Input: part model. Units: mm. Frame: model coordinates. A direction names the side the tool comes from. Round coordinates to 2 decimals unless told otherwise and drop trailing zeros. Write each loop counter-clockwise with the first axis right and the second up, starting at its lowest first coordinate (ties: lowest second). Pieces come first, ordered by that corner, then holes. Notation, with made-up numbers: (-33.75, 75.5) -> (3.25, 75.5) arc R35 cw to (3.25, 107.5) -> close; hole circle Ø5 at (62.5, -38.5). An arc over 180 degrees is marked (long way). Write item = value, one per line. Start each with the question number.
```python
from build123d import *

# Parameters (mm, degrees)
SKETCH1_W           = 11
SKETCH1_H           = 76
BOSS_EXTRUDE1_DEPTH = 7
SKETCH4_R           = 2.5
SKETCH5_W           = 3
SKETCH5_H           = 3
BOSS_EXTRUDE2_DEPTH = 4.5
SKETCH6_W           = 2
SKETCH6_H           = 4
CUT_EXTRUDE2_DEPTH  = 2
BOSS_EXTRUDE3_DEPTH = 3
SKETCH10_W          = 11
SKETCH10_H          = 3.5
CUT_EXTRUDE5_DEPTH  = 35
CUT_EXTRUDE6_REACH  = 41.912
SKETCH11_R          = 2.5
SKETCH12_W          = 11
SKETCH12_H          = 2.25
CUT_EXTRUDE9_DEPTH  = 5
CUT_EXTRUDE10_REACH = 41.58
BOSS_EXTRUDE4_START = 2.5
SKETCH15_R          = 4
SKETCH15_R_2        = 2.5
BOSS_EXTRUDE4_DEPTH = 2.5


with BuildPart() as part:
    # Sketch1 → Boss-Extrude1 (new body)
    with BuildSketch(Plane(origin=(0, 0, 0), x_dir=(1, 0, 0), z_dir=(0, 1, 0))):
        Rectangle(SKETCH1_W, SKETCH1_H)
    extrude(amount=BOSS_EXTRUDE1_DEPTH)

    # Cut-Sweep2: sweep along a path in Sketch3
    with BuildLine(Plane.ZY) as cut_sweep2_path:
        Line((-38, 3.5), (28, 3.5))
        ThreePointArc((28, 3.5), (30.121320344, 2.621320344), (31, 0.5))
        Line((31, 0.5), (31, 0))
    # Sketch4 → Cut-Sweep2 (sweep, cut)
    with BuildSketch(Plane(origin=(0, 0, -38), x_dir=(-1, 0, 0), z_dir=(0, 0, -1))):
        with Locations((0, 3.5)):
            Circle(SKETCH4_R)
    sweep(path=cut_sweep2_path.line, mode=Mode.SUBTRACT)

    # Sketch5 → Boss-Extrude2 (add)
    with BuildSketch(Plane.ZY.offset(5.5)):
        with Locations((31.5, 3.5)):
            Rectangle(SKETCH5_W, SKETCH5_H)
    boss_extrude2 = extrude(amount=BOSS_EXTRUDE2_DEPTH)

    # Mirror1: Boss-Extrude2 across plane
    add(boss_extrude2.mirror(Plane.ZY))

    # Sketch6 → Cut-Extrude2 (cut)
    with BuildSketch(Plane.XY.offset(33)):
        with Locations((-7.25, 4)):
            Rectangle(SKETCH6_W, SKETCH6_H)
    cut_extrude2 = extrude(amount=-CUT_EXTRUDE2_DEPTH, mode=Mode.SUBTRACT)

    # Mirror2: Cut-Extrude2 across plane
    add(cut_extrude2.mirror(Plane.ZY), mode=Mode.SUBTRACT)

    # Sketch7 → Boss-Extrude3 (add)
    with BuildSketch(Plane(origin=(0, 5, 0), x_dir=(1, 0, 0), z_dir=(0, 1, 0))):
        Polygon((-10, -30), (-5.5, -25.5), (-5.5, -30), align=None)
    boss_extrude3 = extrude(amount=-BOSS_EXTRUDE3_DEPTH)

    # Mirror3: Boss-Extrude3 across plane
    add(boss_extrude3.mirror(Plane.ZY))

    # Sketch10 → Cut-Extrude5 (cut)
    with BuildSketch(Plane(origin=(0, 0, -38), x_dir=(-1, 0, 0), z_dir=(0, 0, -1))):
        with Locations((0, 3.5)):
            Rectangle(SKETCH10_W, SKETCH10_H)
    extrude(amount=-CUT_EXTRUDE5_DEPTH, mode=Mode.SUBTRACT)

    # Sketch11 → Cut-Extrude6 (cut, up to next)
    with BuildSketch(Plane(origin=(0, 7, 0), x_dir=(1, 0, 0), z_dir=(0, 1, 0)), mode=Mode.PRIVATE) as cut_extrude6_sk1:
        with Locations(Location((0, 13, 0), (0, 0, 270))):
            Circle(SKETCH11_R)
    cut_extrude6_tool1 = extrude(cut_extrude6_sk1.sketch, amount=-CUT_EXTRUDE6_REACH, mode=Mode.PRIVATE) & part.part
    add(cut_extrude6_tool1.solids().sort_by_distance((0, 7, -13))[0], mode=Mode.SUBTRACT)

    # Sketch12 → Cut-Extrude9 (cut)
    with BuildSketch(Plane.XY.offset(38)):
        with Locations((0, 5.875)):
            Rectangle(SKETCH12_W, SKETCH12_H)
    extrude(amount=-CUT_EXTRUDE9_DEPTH, mode=Mode.SUBTRACT)

    # Sketch14 → Cut-Extrude10 (cut, up to next)
    with BuildSketch(Plane(origin=(0, 4.75, 0), x_dir=(1, 0, 0), z_dir=(0, 1, 0)), mode=Mode.PRIVATE) as cut_extrude10_sk1:
        with BuildLine():
            Line((-2.5, -34.5), (2.5, -34.5))
            ThreePointArc((2.5, -34.5), (3.5, -35.5), (2.5, -36.5))
            Line((2.5, -36.5), (-2.5, -36.5))
            ThreePointArc((-2.5, -36.5), (-3.5, -35.5), (-2.5, -34.5))
        make_face()
    cut_extrude10_tool1 = extrude(cut_extrude10_sk1.sketch, amount=-CUT_EXTRUDE10_REACH, mode=Mode.PRIVATE) & part.part
    add(cut_extrude10_tool1.solids().sort_by_distance((0, 4.75, 35.5))[0], mode=Mode.SUBTRACT)

    # Sketch15 → Boss-Extrude4 (add)
    with BuildSketch(Plane(origin=(0, 7, 0), x_dir=(1, 0, 0), z_dir=(0, 1, 0)).offset(BOSS_EXTRUDE4_START)):
        with Locations(Location((0, 13, 0), (0, 0, 270))):
            Circle(SKETCH15_R)
        with Locations(Location((0, 13, 0), (0, 0, 270))):
            Circle(SKETCH15_R_2, mode=Mode.SUBTRACT)
    extrude(amount=-BOSS_EXTRUDE4_DEPTH)


solid = part.part
```
1. Section A-A (z = -13). Output: boundary loops of the cut face in (x, y).
2. Reachability of faces 1 (the flat face through (0, 2, 36.5)), 2 (the cylindrical face through (-2.4, 8.3, -16.2)), 3 (the flat face through (-4, 1.75, -21)) from +Z, -Z, +X, -X, +Y, -Y: full face, straight path, thin tool, end or side. Return the list, or none.
3. Section B-B (x = 0). Output: boundary loops of the cut face in (y, z).
4. Pin query (flat end, axial travel): P1, Ø4, axis at y = 2, z = -27.5, coming from the +X side; P2, Ø4, axis at x = 4, z = -28.5, coming from the +Y side; P3, Ø5, axis at y = 1, z = 21, coming from the -X side. Return the tip coordinate at first contact, or that it passes through.
5. Section D-D (x = 4.75). Output: boundary loops of the cut face in (y, z).
6. Line query: line 1 along Y through (x, z) = (-5.25, -28); line 2 along X through (y, z) = (8.45, -13); line 3 along Z through (x, y) = (0, 0.4). Output: solid intervals per line, ascending.
7. Mould query, pull axis Y, two halves, no side actions, for faces 4 (the flat face through (4, 4, -3)), 5 (the flat face through (6.25, 3, 32)), 6 (the flat face through (-7, 5, 30)). Classes: pulls with the +Y half, pulls with the -Y half, needs draft (parallel to the pull), parting line crosses it, or undercut.
8. Section C-C (z = -31). Output: boundary loops of the cut face in (x, y), then the cut area to 3 significant figures.
Check sheet entries:
q1.outline = (-5.5, 0) -> (5.5, 0) -> (5.5, 1.75) -> (1.79, 1.75) arc R2.5 cw to (-1.79, 1.75) -> (-5.5, 1.75) -> close; (-5.5, 5.25) -> (-2.5, 5.25) -> (-2.5, 9.5) -> (-4, 9.5) -> (-4, 7) -> (-5.5, 7) -> close; (2.5, 5.25) -> (5.5, 5.25) -> (5.5, 7) -> (4, 7) -> (4, 9.5) -> (2.5, 9.5) -> close
q2.face_1 = +Y, -Y
q2.face_2 = +Y
q2.face_3 = -Z, +X, -X
q3.outline = (0, -38) -> (1, -38) -> (1, 28) arc R0.5 ccw to (0.5, 28.5) -> (0, 28.5) -> close; (0, 33.5) -> (0.5, 33.5) arc R5.5 cw to (6, 28) -> (6, -10.5) -> (9.5, -10.5) -> (9.5, -9) -> (7, -9) -> (7, 33) -> (4.75, 33) -> (4.75, 34.5) -> (0, 34.5) -> close; (0, 36.5) -> (4.75, 36.5) -> (4.75, 38) -> (0, 38) -> close; (6, -38) -> (7, -38) -> (7, -17) -> (9.5, -17) -> (9.5, -15.5) -> (6, -15.5) -> close
q4.P1 = 5.5
q4.P2 = 7
q4.P3 = -5.5
q5.outline = (0, -38) -> (1.75, -38) -> (1.75, -3) -> (5.25, -3) -> (5.25, -38) -> (7, -38) -> (7, 33) -> (4.75, 33) -> (4.75, 38) -> (0, 38) -> close
q6.line_1 = 0 to 1.75, 5.25 to 7
q6.line_2 = -4 to -2.5, 2.5 to 4
q6.line_3 = -38 to 28.5, 33.5 to 34.5, 36.5 to 38
q7.face_4 = undercut
q7.face_5 = needs draft
q7.face_6 = pulls with the +Y half
q8.outline = (-5.5, 0) -> (5.5, 0) -> (5.5, 1.75) -> (1.79, 1.75) arc R2.5 cw to (-1.79, 1.75) -> (-5.5, 1.75) -> close; (-5.5, 5.25) -> (-1.79, 5.25) arc R2.5 cw to (1.79, 5.25) -> (5.5, 5.25) -> (5.5, 7) -> (-5.5, 7) -> close
q8.area = 34.8 mm2
